Geometry: final body of the model. Coordinates: model frame, mm. A direction names the side the tool comes from. Coordinates: 2 decimals unless noted, no trailing zeros. Order: outer loops, then holes, each group sorted by start corner. A loop starts at its lowest first (then second) coordinate and runs counter-clockwise, first axis right, second up. Notation, with made-up numbers: (3, -33) -> (56, -33) arc R25 ccw to (56, -10) -> close; hole circle Ø1 at (-5, 35). An arc over 180 degrees is marked (long way). Use CSV: the item, a comma, the result in double quotes. Start each with the question number.
from build123d import *

# Parameters (mm, degrees)
SKETCH_1_W                         = 626
SKETCH_1_H                         = 70
SM_BASE_FLANGE_1_DEPTH             = 1.5
SM_EDGE_FLANGE_1_STRIP_W           = 7.4732
SM_EDGE_FLANGE_1_STRIP_H           = 1.5
SM_EDGE_FLANGE_1_STRIP_CUT_DEPTH   = 626
SM_EDGE_FLANGE_1_STRIP_2_W         = 7.4732
SM_EDGE_FLANGE_1_STRIP_2_H         = 1.5
SM_EDGE_FLANGE_1_STRIP_CUT_2_DEPTH = 626
SM_EDGE_FLANGE_1_DEPTH             = 626
SM_EDGE_FLANGE_1_BEND_DEPTH        = 626
SKETCH_8_W                         = 2
SKETCH_8_H                         = 4.5
SM_BASE_FLANGE_1_2_DEPTH           = 1.5
CUT_EXTRUDE_1_REACH                = 319.478
SKETCH_11_W                        = 10
SKETCH_11_H                        = 2.2366
SM_BASE_FLANGE_2_DEPTH             = 1.5
SKETCH_13_R                        = 3.25
CUT_EXTRUDE_2_DEPTH                = 1.5


# Sheet-metal steps are written as plain solids
with BuildPart() as part:
    # Sketch 1 → Sm Base Flange 1 (new body)
    with BuildSketch(Plane.XY):
        Rectangle(SKETCH_1_W, SKETCH_1_H)
    extrude(amount=-SM_BASE_FLANGE_1_DEPTH)

    # Ребро-кромка1 strip (across the edge) → Ребро-кромка1 strip cut (cut)
    with BuildSketch(Plane(origin=(313, 35, 0), x_dir=(0, -1, 0), z_dir=(-1, 0, 0))):
        with Locations((-1.5, -0.75)):
            Rectangle(SM_EDGE_FLANGE_1_STRIP_W, SM_EDGE_FLANGE_1_STRIP_H)
    extrude(amount=SM_EDGE_FLANGE_1_STRIP_CUT_DEPTH, mode=Mode.SUBTRACT)

    # Ребро-кромка1 strip 2 (across the edge) → Ребро-кромка1 strip cut 2 (cut)
    with BuildSketch(Plane(origin=(-313, -35, 0), x_dir=(0, 1, 0), z_dir=(1, 0, 0))):
        with Locations((-1.5, -0.75)):
            Rectangle(SM_EDGE_FLANGE_1_STRIP_2_W, SM_EDGE_FLANGE_1_STRIP_2_H)
    extrude(amount=SM_EDGE_FLANGE_1_STRIP_CUT_2_DEPTH, mode=Mode.SUBTRACT)

    # Ребро-кромка1 section (across the edge) → Ребро-кромка1 (add)
    with BuildSketch(Plane(origin=(313, 35, 0), x_dir=(0, -1, 0), z_dir=(-1, 0, 0))):
        with BuildLine():
            Line((0, 0.7366), (0, 17))
            Line((0, 17), (1.5, 17))
            Line((1.5, 17), (1.5, 0.7366))
            ThreePointArc((1.5, 0.7366), (1.715745145, 0.215745145), (2.2366, 0))
            Line((2.2366, 0), (2.2366, -1.5))
            ThreePointArc((2.2366, -1.5), (0.655084973, -0.844915027), (0, 0.7366))
        make_face()
    extrude(amount=SM_EDGE_FLANGE_1_DEPTH)

    # Ребро-кромка1 section 2 (across the edge) → Ребро-кромка1 bend (add)
    with BuildSketch(Plane(origin=(-313, -35, 0), x_dir=(0, 1, 0), z_dir=(1, 0, 0))):
        with BuildLine():
            Line((0, 0.7366), (0, 17))
            Line((0, 17), (1.5, 17))
            Line((1.5, 17), (1.5, 0.7366))
            ThreePointArc((1.5, 0.7366), (1.715745145, 0.215745145), (2.2366, 0))
            Line((2.2366, 0), (2.2366, -1.5))
            ThreePointArc((2.2366, -1.5), (0.655084973, -0.844915027), (0, 0.7366))
        make_face()
    extrude(amount=SM_EDGE_FLANGE_1_BEND_DEPTH)

    # Эскиз8 → Sm Base Flange 1 2 (add)
    with BuildSketch(Plane.XY):
        with Locations((-314, 0)):
            Rectangle(SKETCH_8_W, SKETCH_8_H)
        with Locations((314, 0)):
            Rectangle(SKETCH_8_W, SKETCH_8_H)
    extrude(amount=-SM_BASE_FLANGE_1_2_DEPTH)

    # Эскиз11 → Вырез-Вытянуть1 (cut, up to next)
    with BuildSketch(Plane.XY.offset(17), mode=Mode.PRIVATE) as cut_extrude_1_sk1:
        with Locations((-308, 33.8817)):
            Rectangle(SKETCH_11_W, SKETCH_11_H)
    cut_extrude_1_tool1 = extrude(cut_extrude_1_sk1.sketch, amount=-CUT_EXTRUDE_1_REACH, mode=Mode.PRIVATE) & part.part
    # Эскиз11 → Вырез-Вытянуть1 (cut, up to next)
    with BuildSketch(Plane.XY.offset(17), mode=Mode.PRIVATE) as cut_extrude_1_sk2:
        with Locations((-308, -33.8817)):
            Rectangle(SKETCH_11_W, SKETCH_11_H)
    cut_extrude_1_tool2 = extrude(cut_extrude_1_sk2.sketch, amount=-CUT_EXTRUDE_1_REACH, mode=Mode.PRIVATE) & part.part
    # Эскиз11 → Вырез-Вытянуть1 (cut, up to next)
    with BuildSketch(Plane.XY.offset(17), mode=Mode.PRIVATE) as cut_extrude_1_sk3:
        with Locations((308, -33.8817)):
            Rectangle(SKETCH_11_W, SKETCH_11_H)
    cut_extrude_1_tool3 = extrude(cut_extrude_1_sk3.sketch, amount=-CUT_EXTRUDE_1_REACH, mode=Mode.PRIVATE) & part.part
    # Эскиз11 → Вырез-Вытянуть1 (cut, up to next)
    with BuildSketch(Plane.XY.offset(17), mode=Mode.PRIVATE) as cut_extrude_1_sk4:
        with Locations((308, 33.8817)):
            Rectangle(SKETCH_11_W, SKETCH_11_H)
    cut_extrude_1_tool4 = extrude(cut_extrude_1_sk4.sketch, amount=-CUT_EXTRUDE_1_REACH, mode=Mode.PRIVATE) & part.part
    add(cut_extrude_1_tool1.solids().sort_by_distance((-308, 33.8817, 17))[0], mode=Mode.SUBTRACT)
    add(cut_extrude_1_tool2.solids().sort_by_distance((-308, -33.8817, 17))[0], mode=Mode.SUBTRACT)
    add(cut_extrude_1_tool3.solids().sort_by_distance((308, -33.8817, 17))[0], mode=Mode.SUBTRACT)
    add(cut_extrude_1_tool4.solids().sort_by_distance((308, 33.8817, 17))[0], mode=Mode.SUBTRACT)

    # Эскиз12 → Выступ2 (add)
    with BuildSketch(Plane.XY):
        Polygon((-313, 32.7634), (-313, 41.7634), (-310, 41.7634), (-303.5, 35.2634), (-303.5, 32.7634), align=None)
        Polygon((-303.5, -32.7634), (-313, -32.7634), (-313, -41.7634), (-310, -41.7634), (-303.5, -35.2634), align=None)
        Polygon((313, -32.7634), (313, -41.7634), (310, -41.7634), (303.5, -35.2634), (303.5, -32.7634), align=None)
        Polygon((303.5, 32.7634), (313, 32.7634), (313, 41.7634), (310, 41.7634), (303.5, 35.2634), align=None)
    extrude(amount=-SM_BASE_FLANGE_2_DEPTH)

    # Эскиз13 → Вырез-Вытянуть2 (cut)
    with BuildSketch(Plane.XY):
        with Locations((-270, 22)):
            Circle(SKETCH_13_R)
        with Locations((-222, 22)):
            Circle(SKETCH_13_R)
        with Locations(Location((222, 22, 0), (0, 0, 180))):
            Circle(SKETCH_13_R)
        with Locations(Location((270, 22, 0), (0, 0, 180))):
            Circle(SKETCH_13_R)
    extrude(amount=-CUT_EXTRUDE_2_DEPTH, mode=Mode.SUBTRACT)


solid = part.part
(1) Section B-B (x = -174). Return loops of the section in (y, z).
(2) First-contact query: pin 1 (1.8 mm diameter, centred on y = 33.5, z = 5.5, fed in from -X); pin 2 (3 mm diameter, centred on x = -23.5, z = 2, fed in from +Y); pin 3 (0.8 mm diameter, centred on y = 34, z = -1, fed in from -X). Flat tips, straight axial feed; report the tip coordinate or a pass-through.
(3) Section A-A (z = 4.75). Return loops of the section in (x, y).
(4) Access query for faces 1 (the face through (-4, -33.5, 9)), 2 (the face through (4, 35, 9)). Directions: +Z, -Z, +X, -X, +Y, -Y. A direction counts if a zero-diameter tool reaches every point of the face in a straight line with its end or side. Return the directions, or none.
(5) Line query: line 1 (Y direction, x = 2, z = 9.75); line 2 (Z direction, x = -40, y = 21); line 3 (X direction, y = -16, z = -0.25). Output: solid intervals per line, ascending. Write a range as from..to.
(6) Section C-C (y = 13.5). Return loops of the section in (x, z), then the cut area to 3 significant figures.
(7) Mould query, pull axis Y, two halves, no side actions, for faces 3 (the face through (4, 33.5, 9)), 4 (the face through (-4, -35, 9)), 5 (the face through (4, 1, -1.5)). Classes: pulls with the +Y half, pulls with the -Y half, needs draft (parallel to the pull), parting line crosses it, or undercut.
Check sheet entries:
1,outline,"(-35, 0.74) arc R2.24 ccw to (-32.76, -1.5) -> (32.76, -1.5) arc R2.24 ccw to (35, 0.74) -> (35, 17) -> (33.5, 17) -> (33.5, 0.74) arc R0.74 cw to (32.76, 0) -> (-32.76, 0) arc R0.74 cw to (-33.5, 0.74) -> (-33.5, 17) -> (-35, 17) -> close"
2,pin 1,"stops at x = -303"
2,pin 2,"stops at y = 35"
2,pin 3,"stops at x = -313"
3,outline,"(-303, -35) -> (303, -35) -> (303, -33.5) -> (-303, -33.5) -> close; (-303, 33.5) -> (303, 33.5) -> (303, 35) -> (-303, 35) -> close"
4,face 1,"+Z, +X, -X"
4,face 2,"+Z, -Z, +X, -X, +Y"
5,line 1,"y = -35..-33.5, 33.5..35"
5,line 2,"z = -1.5..0"
5,line 3,"x = -313..313"
6,outline,"(-313, -1.5) -> (313, -1.5) -> (313, 0) -> (-313, 0) -> close"
6,area,"939 mm^2"
7,face 3,"undercut"
7,face 4,"pulls with the -Y half"
7,face 5,"needs draft"
